For this review, take the finished solid that the model builds, in its own axes (mm). A direction names the side the tool comes from. Give positions to 0.01 mm unless a question says otherwise; leave off trailing zeros. Loops run counter-clockwise (first coordinate to the right, second up) from the corner with the lowest first, then second, coordinate; pieces in that order, holes last. Notation, with made-up numbers: (17, 64.25) - (64, 64.25) arc R27 cw to (64, 101.25) - close; hole circle Ø7 at (-36.75, -23.75). An arc over 180 degrees is marked (long way). Put each result on its own line as item: value. Start each with the question number.
from build123d import *

# Parameters (mm, degrees)
SKETCH_W        = 30
SKETCH_H        = 75
PAD_DEPTH       = 20
POCKET_DEPTH    = 30.001
POCKET001_DEPTH = 30.001
SKETCH003_R     = 1.8
POCKET002_DEPTH = 18.001
SKETCH004_W     = 22
SKETCH004_H     = 10
POCKET003_DEPTH = 75.001
SKETCH005_W     = 1.992782
SKETCH005_H     = 16
SKETCH005_W_2   = 2
PAD001_DEPTH    = 2.5
FILLET_R        = 1
CHAMFER_SIZE    = 1


with BuildPart() as part:
    # Sketch → Pad (new body)
    with BuildSketch(Plane.XY):
        with Locations((0, 50.5)):
            Rectangle(SKETCH_W, SKETCH_H)
    extrude(amount=PAD_DEPTH)

    # Sketch001 → Pocket (cut, through all)
    with BuildSketch(Plane(origin=(-15, 0, 0), x_dir=(0, -1, 0), z_dir=(-1, 0, 0))):
        Polygon((-90.237335, 21), (-17.197588, 21), (-21.197588, 4), (-90.237335, 4), align=None)
    extrude(amount=-POCKET_DEPTH, mode=Mode.SUBTRACT)

    # Sketch002 → Pocket001 (cut, through all)
    with BuildSketch(Plane(origin=(-15, 0, 0), x_dir=(0, -1, 0), z_dir=(-1, 0, 0))):
        with BuildLine():
            ThreePointArc((-13.300504, 16.341381), (-14.741789, 17.980276), (-16.608656, 16.849752))
            Line((-16.608656, 16.849752), (-21.00001, 4))
            Line((-25, 4), (-21.00001, 4))
            Line((-25, 18.137928), (-25, 4))
            Line((-25, 18.137928), (-12.210917, 22))
            Line((-12.210917, 22), (-13, 4))
            Line((-13, 4), (-13.300504, 16.341381))
        make_face()
    extrude(amount=-POCKET001_DEPTH, mode=Mode.SUBTRACT)

    # Sketch003 → Pocket002 (cut, through all)
    with BuildSketch(Plane(origin=(0, 0, 0), x_dir=(1, 0, 0), z_dir=(0, 0, -1))):
        with Locations((0, -80)):
            Circle(SKETCH003_R)
        with Locations((0, -70)):
            Circle(SKETCH003_R)
        with Locations((0, -60)):
            Circle(SKETCH003_R)
        with Locations((0, -50)):
            Circle(SKETCH003_R)
        with Locations((0, -40)):
            Circle(SKETCH003_R)
        with Locations((0, -30)):
            Circle(SKETCH003_R)
    extrude(amount=-POCKET002_DEPTH, mode=Mode.SUBTRACT)

    # Sketch004 → Pocket003 (cut, through all)
    with BuildSketch(Plane.XZ.offset(-13)):
        with Locations((0, 15)):
            Rectangle(SKETCH004_W, SKETCH004_H)
    extrude(amount=-POCKET003_DEPTH, mode=Mode.SUBTRACT)

    # Sketch005 → Pad001 (new body)
    with BuildSketch(Plane.XY.offset(4)):
        with Locations((-13.996391, 80)):
            Rectangle(SKETCH005_W, SKETCH005_H)
        with Locations((14, 80)):
            Rectangle(SKETCH005_W_2, SKETCH005_H)
    extrude(amount=PAD001_DEPTH)

    # Fillet
    fillet_edges = [part.edges().sort_by_distance(p)[0] for p in [
        (-13.996391, 72, 6.5),
        (14, 72, 6.5),
        (14, 88, 6.5),
        (-13.996391, 88, 6.5),
    ]]
    fillet(fillet_edges, radius=FILLET_R)

    # Chamfer
    chamfer_edges = [part.edges().sort_by_distance(p)[0] for p in [
        (0, 13, 0),
        (15, 50.5, 0),
        (-15, 50.5, 0),
        (0, 88, 0),
    ]]
    chamfer(chamfer_edges, length=CHAMFER_SIZE)


solid = part.part
1) Take a section at B-B on z = 11.75. State the section outline as (x, y) points, and give its area (3 significant figures).
2) Take a section at D-D on y = 24. State the section outline as (x, z) points.
3) Mouldability with a two-part tool opening along Y and no side actions: class faces 5 (the flat face through (14, 80, 6.5)), 6 (the flat face through (-14, 72, 5)), 7 (the cylindrical face through (-13, 15, 18)), 8 (the flat face through (0, 13, 2)) as released by +Y, released by -Y, zero draft, split by the parting line, or undercut.
4) Take a section at C-C on x = 5. State the section outline as (y, z) points, and give its area (3 significant figures).
5) Machinability: for faces 1 (the flat face through (0, 16, 10)), 2 (the flat face through (-14, 80, 6.5)), 3 (the flat face through (14, 72, 5)), 4 (the flat face through (0, 88, 3)), which of the approach directions +Z, -Z, +X, -X, +Y, -Y give a long, thin tool a straight path to every point of the face, cutting with its end or side? Answer none if there is none.
6) Insertion check: P1, Ø6.5, axis at x = 1.5, y = 15, coming from the +Z side; P2, Ø2, axis at x = 14, y = 78, coming from the +Z side; P3, Ø3, axis at x = 0, y = 60, coming from the -Z side; P4, Ø4, axis at x = 0, y = 70, coming from the +Z side. Each pin has a flat end and moves straight along its axis. Give the tip position at first contact, or say it passes through.
7) Wall thickness on probe 1 along X at (y, z) = (30, 1.15); probe 2 along Z at (x, y) = (3, 52.5); probe 3 along Y at (x, z) = (8, 5): over which ranges is each line inside the solid? List them lowest first.
Answers follow:
1. outline: (-15, 13.19) - (-11, 13.19) - (-11, 18.35) - (-15, 18.35) - close; (11, 13.19) - (15, 13.19) - (15, 18.35) - (11, 18.35) - close
1. area: 41.3 mm2
2. outline: (-15, 1) - (-14, 0) - (14, 0) - (15, 1) - (15, 4) - (-15, 4) - close
3. face 5: zero draft
3. face 6: undercut
3. face 7: split by the parting line
3. face 8: released by -Y
4. outline: (13, 1) - (14, 0) - (87, 0) - (88, 1) - (88, 4) - (21, 4) - (18.95, 10) - (13.15, 10) - (13, 4) - close
4. area: 340 mm2
5. face 1: +Z, +Y, -Y
5. face 2: +Z, +X, -X, +Y
5. face 3: +Z, +X, -X
5. face 4: +Z, -Z, +X, -X, +Y
6. P1: z = 10
6. P2: z = 6.5
6. P3: through
6. P4: z = 4
7. probe 1: -15 to -1.8, 1.8 to 15
7. probe 2: 0 to 4
7. probe 3: 13.02 to 20.66
